Work out the finished part from the listing and answer in its coordinate system (mm). Face numbers are marked on the shaded views. A direction names the side the tool comes from. Round coordinates to 2 decimals unless told otherwise and drop trailing zeros. Order: outer loops, then holes, each group sorted by start corner. A loop starts at its lowest first (then second) coordinate and runs counter-clockwise, first axis right, second up. Notation, with made-up numbers: (3.5, 11) -> (49.5, 11) arc R20 cw to (49.5, 45) -> close; hole circle Ø4 at (16, 17). An arc over 180 degrees is marked (long way). Use one line per item in the form item = value.
```python
from build123d import *

# Parameters (mm, degrees)
F0_W     = 74.1118490696
F0_H     = 45.0000055134
F1_DEPTH = 5
F3_W     = 38.6348655447
F3_H     = 16.8519383296
F4_DEPTH = 17.7
F5_R     = 5


with BuildPart() as f1:
    # F0 (on Top) → F1 (new body)
    with BuildSketch(Plane.XY):
        with Locations((37.0559245348, 22.5000027567)):
            Rectangle(F0_W, F0_H)
    extrude(amount=F1_DEPTH)

    # F3 (on face) → F4 (join)
    with BuildSketch(Plane.XY.offset(5)):
        with Locations((29.2525482364, 21.4091469534)):
            Rectangle(F3_W, F3_H)
    extrude(amount=F4_DEPTH)

    # F5
    f5_edges = [f1.edges().sort_by_distance(p)[0] for p in [
        (48.569981, 12.983178, 13.85),
        (48.569981, 29.835116, 13.85),
        (48.569981, 21.409147, 5),
        (48.569981, 21.409147, 22.7),
        (29.252548, 12.983178, 5),
        (29.252548, 29.835116, 5),
    ]]
    fillet(f5_edges, radius=F5_R)


solid = f1.part
```
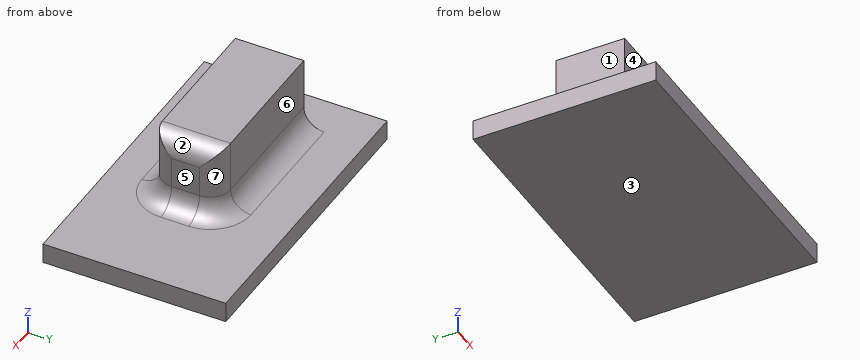
Item 1: The part is cut by section B-B, the plane y = 23.5. Give the vertices of the cut face in (x, z).
Findings:
outline = (0, 0) -> (74.11, 0) -> (74.11, 5) -> (53.57, 5) arc R5 cw to (48.57, 10) -> (48.57, 17.7) arc R5 ccw to (43.57, 22.7) -> (9.94, 22.7) -> (9.94, 5) -> (0, 5) -> close
Item 2: The part is cut by section A-A, the plane x = 19. Give the vertices of the cut face in (y, z).
Findings:
outline = (0, 0) -> (45, 0) -> (45, 5) -> (34.84, 5) arc R5 cw to (29.84, 10) -> (29.84, 22.7) -> (12.98, 22.7) -> (12.98, 10) arc R5 cw to (7.98, 5) -> (0, 5) -> close
Item 3: For the marked faces 4, 5, 6 and 7, determine the directions among +Z, -Z, +X, -X, +Y, -Y from which every point of the face is accessible in a straight line to the end or side of a thin tool.
Findings:
face_4 = +Z, +X, -X, -Y
face_5 = +Z, +X, +Y, -Y
face_6 = +Z, +X, -X, +Y
face_7 = +Z, +X, +Y
Item 4: The part is cut by section C-C, the plane z = 19.75. Give the vertices of the cut face in (x, y).
Findings:
outline = (9.94, 12.98) -> (43.57, 12.98) arc R5 ccw to (48.13, 15.93) -> (48.13, 26.89) arc R5 ccw to (43.57, 29.84) -> (9.94, 29.84) -> close
Item 5: Consider line 1 along Z through (x, y) = (64, 2); line 2 along X through (y, z) = (25, 17.25); line 3 along Y through (x, z) = (16, 15). Determine where each line is inside the solid, lowest interval first.
Findings:
line_1 = 0 to 5
line_2 = 9.94 to 48.57
line_3 = 12.98 to 29.84
Item 6: Determine the mould class of the marked faces 1, 2 and 3 for opening direction X: released by +X, released by -X, zero draft, split by the parting line, or undercut.
Findings:
face_1 = released by -X
face_2 = released by +X
face_3 = zero draft
Item 7: Flat-ended cylindrical pins translate along their axes: P1, Ø1.5, axis at x = 13.5, z = 13, coming from the +Y side; P2, Ø12, axis at y = 6, z = 4.5, coming from the -X side; P3, Ø10, axis at x = 23.5, z = 16, coming from the -Y side; P4, Ø2, axis at y = 37, z = 7, coming from the +X side. Find the tip coordinate at first contact, or state that the pin passes through.
Findings:
P1 = 29.84
P2 = 0
P3 = 12.98
P4 = through
Item 8: The part is cut by section D-D, the plane x = 62. Give the vertices of the cut face in (y, z), and give its area (3 significant figures).
Findings:
outline = (0, 0) -> (45, 0) -> (45, 5) -> (0, 5) -> close
area = 225 mm^2
